The figure shows three views and two pictorial views of one solid part (mm, origin at its lowest corner). Answer the questions. A direction names the side the tool comes from. Coordinates: 2 decimals unless noted, no trailing zeros. Order: outer loops, then holes, each group sorted by start corner. A loop starts at its lowest first (then second) coordinate and runs counter-clockwise, first axis right, second up. Notation, with made-up numbers: (6.25, 60) - (20.25, 60) arc R11 ccw to (20.25, 81) - close; hole circle Ø11 at (72, 62.5). An arc over 180 degrees is marked (long way). Use one line per item in the form item = value.
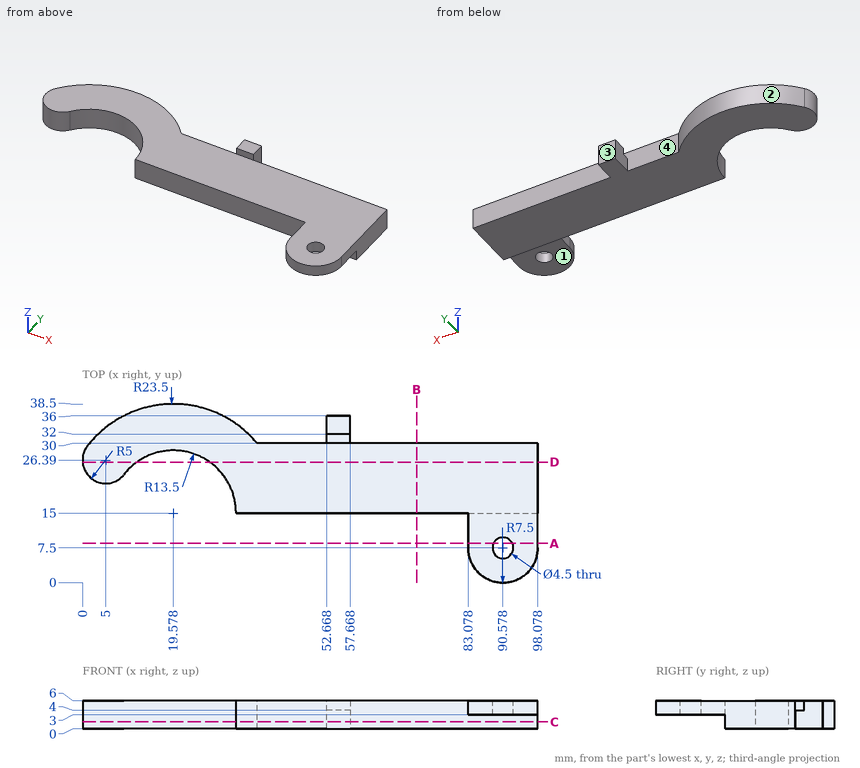
(1) Which of the six approach directions +Z, -Z, +X, -X, +Y, -Y give full straight-line access (tool end or side, diameter ignored) to the marked faces 1 and 2?
Answer list:
face_1 = -Z, +X, -X, -Y
face_2 = +Z, -Z, +Y
(2) Section B-B, the plane x = 72 is taken. Write down the section's boundary in (y, z).
Answer list:
outline = (15, 0) - (30, 0) - (30, 6) - (15, 6) - close
(3) Section A-A, the plane y = 8.5 is taken. Write down the section's boundary in (x, z), then the cut area to 3 significant figures.
Answer list:
outline = (83.08, 3) - (88.56, 3) - (88.56, 6) - (83.08, 6) - close; (92.59, 3) - (98.08, 3) - (98.08, 6) - (92.59, 6) - close
area = 32.9 mm2
(4) Given pin 1 Ø4.5 at (x, y) = (91.5, 6) entering from -Z; pin 2 Ø0.9 at (y, z) = (11, 4.5) entering from -X; pin 3 Ø1.8 at (y, z) = (32, 4) entering from +X; pin 4 Ø4 at (x, y) = (90.58, 7.5) entering from +Z, each flat-ended and moving along its own axis, determine where each tip first touches the part or whether it passes through.
Answer list:
pin_1 = 3
pin_2 = 83.08
pin_3 = 57.67
pin_4 = through
(5) Straight lines are drawn through the part: L1, parallel to X at y = 7.5, z = 5.4; L2, parallel to Y at x = 39.5, z = 2.85; L3, parallel to Y at x = 54.5, z = 0.4. For each, find the intervals that lie inside material, in ascending order.
Answer list:
L1 = 83.08 to 88.33, 92.83 to 98.08
L2 = 15 to 30
L3 = 15 to 36
(6) Section C-C, the plane z = 1.45 is taken. Write down the section's boundary in (x, y).
Answer list:
outline = (1.06, 29.47) arc R5 ccw to (8.94, 23.31) arc R13.5 cw to (33.08, 15) - (98.08, 15) - (98.08, 30) - (57.67, 30) - (57.67, 36) - (52.67, 36) - (52.67, 30) - (37.67, 30) arc R23.5 ccw to start
(7) The mould has two halves that part along X. Classify the marked faces 3 and 4: +X half, -X half, draft (parallel to the pull), parting line (faces both ways), or undercut.
Answer list:
face_3 = draft
face_4 = undercut
(8) Section D-D, the plane y = 26 is taken. Write down the section's boundary in (x, z).
Answer list:
outline = (0.02, 0) - (11.75, 0) - (11.75, 6) - (0.02, 6) - close; (27.4, 0) - (98.08, 0) - (98.08, 6) - (27.4, 6) - close
